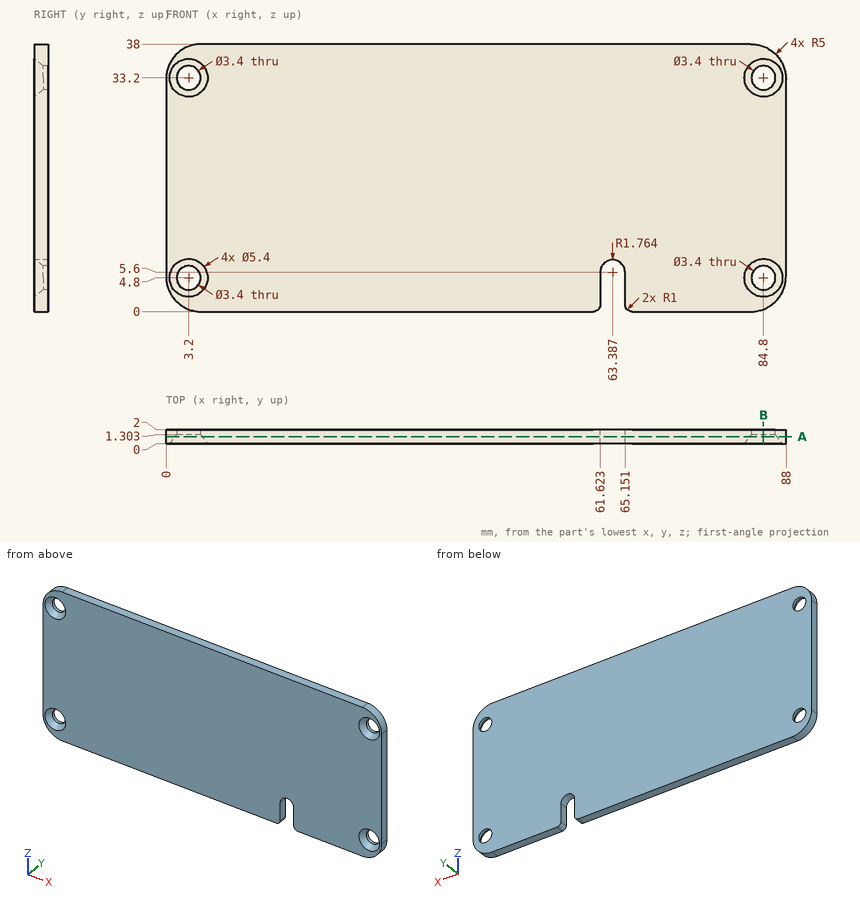
Geometry: see drawing. Coordinates: mm, zero at the bounding-box minimum. Give positions to 0.01 mm unless a question says otherwise; leave off trailing zeros. Loops run counter-clockwise (first coordinate to the right, second up) from the corner with the lowest first, then second, coordinate; pieces in that order, holes last. Notation, with made-up numbers: M -1,72 L 31,72 A38 cw 31,111 Z; hole C 17.5,14.5 d11. An arc over 180 degrees is marked long. Use one line per item in the form item = value.
1. Line query: L1, parallel to X at y = 1.95, z = 33.2; L2, parallel to Z at x = 84.8, y = 1.8 (1 decimal); L3, parallel to X at y = 1.2, z = 32 (1 decimal). Output: solid intervals per line, ascending.
Numbers:
L1 = 0 to 1.5, 4.9 to 83.1, 86.5 to 88
L2 = 0.3 to 3.1, 6.5 to 31.5, 34.9 to 37.7
L3 = 0 to 1.9, 4.5 to 83.5, 86.1 to 88
2. Section query A-A, the plane y = 1. Return the cut outline in (x, z) (1 decimal).
Numbers:
outline = M 0,5 A5 ccw 5,0 L 60.6,0 A1 ccw 61.6,1 L 61.6,5.6 A1.8 cw 65.2,5.6 L 65.2,1 A1 ccw 66.2,0 L 83,0 A5 ccw 88,5 L 88,33 A5 ccw 83,38 L 5,38 A5 ccw 0,33 Z; hole C 3.2,4.8 d3.9; hole C 3.2,33.2 d3.9; hole C 84.8,4.8 d3.9; hole C 84.8,33.2 d3.9
3. Section query B-B, the plane x = 84.8. Return the cut outline in (y, z) (1 decimal).
Numbers:
outline = M 0,0.3 L 2,0.3 L 2,3.1 L 1.3,3.1 L 0,2.1 Z; M 0,7.5 L 1.3,6.5 L 2,6.5 L 2,31.5 L 1.3,31.5 L 0,30.5 Z; M 0,35.9 L 1.3,34.9 L 2,34.9 L 2,37.7 L 0,37.7 Z
4. First-contact query: pin 1 (1 mm diameter, centred on y = 1, z = 2.5, fed in from -X); pin 2 (2.5 mm diameter, centred on x = 84.8, z = 33.2, fed in from -Y). Flat tips, straight axial feed; report the tip coordinate or a pass-through.
Numbers:
pin_1 = 0.42
pin_2 = through
